Can you work these out from the model? Positions are in its coordinate system, mm. Round coordinates to 2 decimals unless told otherwise and drop trailing zeros. Write each loop counter-clockwise with the first axis right and the second up, starting at its lowest first coordinate (ties: lowest second). Pieces come first, ordered by that corner, then holes. Notation, with made-up numbers: M 64,11.5 L 98,11.5 A24 cw 98,27.5 Z; hole C 62,76.25 d11. An arc over 180 degrees is marked long. Answer as a JSON object with one key per item and string values. Group by question number.
1) Suppose I cut it at B-B, the plane z = 8.5. Write out the boundary of the cut face in (x, y), and give its area (3 significant figures).
2) Suppose I cut it at A-A, the plane y = -158.5. Write out the boundary of the cut face in (x, z) (3 decimals), and give its area (3 significant figures).
3) Please list where these lines run through material, in increasing order: L1, parallel to Y at x = 121, z = 25.5; L2, parallel to X at y = -161.5, z = 24.5. Write a range as [from, to].
from build123d import *

# Parameters (mm, degrees)
F0_W     = 762
F0_H     = 2133.6
F1_DEPTH = 28.575
F3_DEPTH = 31.75
F4_DEPTH = 304.8


with BuildPart() as f1:
    # F0 (on Top) → F1 (new body)
    with BuildSketch(Plane.XY):
        Rectangle(F0_W, F0_H)
    extrude(amount=F1_DEPTH)

    # F2 (on face) → F3 (cut)
    with BuildSketch(Plane.XY.offset(28.575)):
        Polygon((12.7, 63.5), (12.7, -76.2), (12.7, -215.9), (139.7, -215.9), (139.7, 63.5), align=None)
    extrude(amount=-F3_DEPTH, mode=Mode.SUBTRACT)

    # F4 (add): a face of the model
    f4_faces = [f1.faces().sort_by_distance(p)[0] for p in [
        (0, -1066.8, 14.2875),
    ]]
    extrude(f4_faces, amount=F4_DEPTH)


solid = f1.part
Results:
{
 "1": {"outline": "M -381,-1371.6 L 381,-1371.6 L 381,1066.8 L -381,1066.8 Z; hole M 12.7,-215.9 L 139.7,-215.9 L 139.7,63.5 L 12.7,63.5 Z", "area": "1,820,000 mm^2"},
 "2": {"outline": "M -381,0 L 12.7,0 L 12.7,28.575 L -381,28.575 Z; M 139.7,0 L 381,0 L 381,28.575 L 139.7,28.575 Z", "area": "18,100 mm^2"},
 "3": {"L1": "[-1371.6, -215.9], [63.5, 1066.8]", "L2": "[-381, 12.7], [139.7, 381]"}
}
